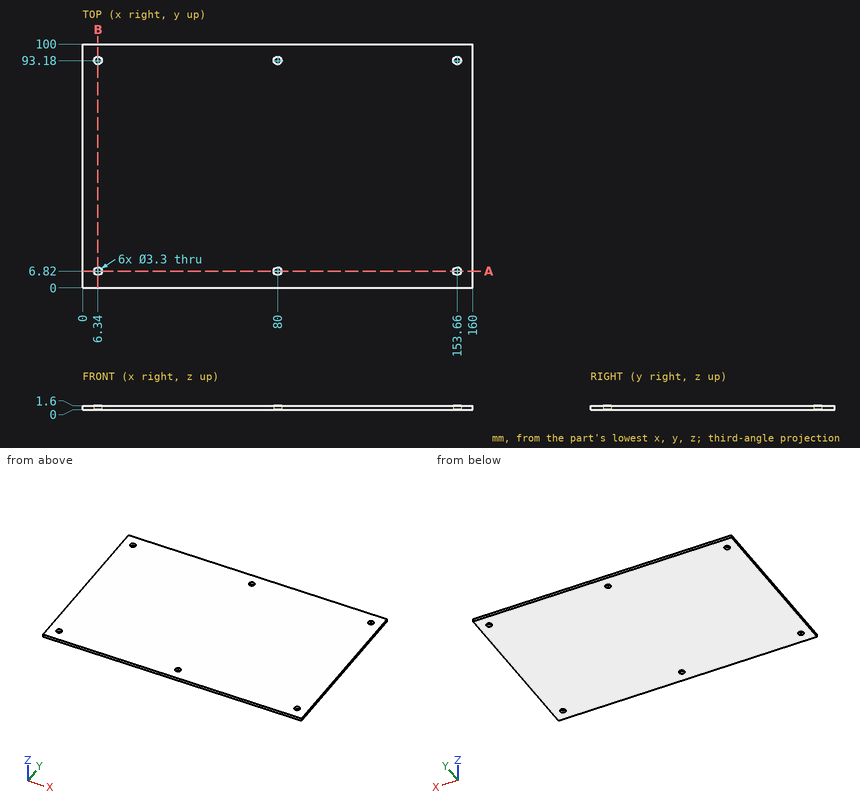
Part print with two shaded views. Sizes in mm from the minimum x, y, z corner. Round coordinates to 2 decimals unless told otherwise and drop trailing zeros. Order: outer loops, then holes, each group sorted by start corner. A loop starts at its lowest first (then second) coordinate and runs counter-clockwise, first axis right, second up. Notation, with made-up numbers: M 22.5,46 L 49.5,46 A24 cw 49.5,71 Z; hole C -21.75,-9.5 d10. An arc over 180 degrees is marked long. Use CSV: the item, a comma, the result in double quotes.
Item 1: Saw through at B-B (x = 6.34). List the corners of the cut face in (y, z), plus the area to 3 significant figures.
Worked answers:
outline,"M 0,0 L 5.17,0 L 5.17,1.6 L 0,1.6 Z; M 8.47,0 L 91.53,0 L 91.53,1.6 L 8.47,1.6 Z; M 94.83,0 L 100,0 L 100,1.6 L 94.83,1.6 Z"
area,"149 mm²"
Item 2: Probe probe 1 along X at (y, z) = (93.18, 0.4); probe 2 along Y at (x, z) = (153.66, 1.35); probe 3 along X at (y, z) = (7.5, 0.55). List the from-to ranges inside material, lowest first.
Worked answers:
probe 1,"0 to 4.69, 7.99 to 78.35, 81.65 to 152.01, 155.31 to 160"
probe 2,"0 to 5.17, 8.47 to 91.53, 94.83 to 100"
probe 3,"0 to 4.84, 7.84 to 78.5, 81.5 to 152.16, 155.16 to 160"
Item 3: Saw through at A-A (y = 6.82). List the corners of the cut face in (x, z), plus the area to 3 significant figures.
Worked answers:
outline,"M 0,0 L 4.69,0 L 4.69,1.6 L 0,1.6 Z; M 7.99,0 L 78.35,0 L 78.35,1.6 L 7.99,1.6 Z; M 81.65,0 L 152.01,0 L 152.01,1.6 L 81.65,1.6 Z; M 155.31,0 L 160,0 L 160,1.6 L 155.31,1.6 Z"
area,"240 mm²"
